Geometry check sheet. Reference: the model listing, model coordinates, mm. A direction names the side the tool comes from. Round coordinates to 2 decimals unless told otherwise and drop trailing zeros. Write each loop counter-clockwise with the first axis right and the second up, starting at its lowest first coordinate (ties: lowest second). Pieces come first, ordered by that corner, then holes. Notation, with made-up numbers: (-18, -13) -> (15, -13) arc R23 ccw to (15, 16) -> close; hole circle Ø3 at (-39, 32.25). An arc over 180 degrees is marked (long way). Use a Markdown table: item, result.
```python
from build123d import *

# Parameters (mm, degrees)
SKETCH1_W           = 85
SKETCH1_H           = 20
BOSS_EXTRUDE1_DEPTH = 5
CUT_EXTRUDE1_REACH  = 7
SKETCH2_W           = 8
SKETCH2_H           = 5.2


with BuildPart() as part:
    # Sketch1 → Boss-Extrude1 (new body)
    with BuildSketch(Plane.XY):
        with Locations((20.528766582, 10)):
            Rectangle(SKETCH1_W, SKETCH1_H)
    extrude(amount=BOSS_EXTRUDE1_DEPTH)

    # Sketch2 → Cut-Extrude1 (cut, up to next)
    with BuildSketch(Plane.XY.offset(5), mode=Mode.PRIVATE) as cut_extrude1_sk1:
        with Locations((-7.971233418, 4.6)):
            Rectangle(SKETCH2_W, SKETCH2_H)
    cut_extrude1_tool1 = extrude(cut_extrude1_sk1.sketch, amount=-CUT_EXTRUDE1_REACH, mode=Mode.PRIVATE) & part.part
    add(cut_extrude1_tool1.solids().sort_by_distance((-7.971233, 4.6, 5))[0], mode=Mode.SUBTRACT)
    # Sketch2 → Cut-Extrude1 (cut, up to next)
    with BuildSketch(Plane.XY.offset(5), mode=Mode.PRIVATE) as cut_extrude1_sk2:
        with Locations((11.028766582, 4.6)):
            Rectangle(SKETCH2_W, SKETCH2_H)
    cut_extrude1_tool2 = extrude(cut_extrude1_sk2.sketch, amount=-CUT_EXTRUDE1_REACH, mode=Mode.PRIVATE) & part.part
    add(cut_extrude1_tool2.solids().sort_by_distance((11.028767, 4.6, 5))[0], mode=Mode.SUBTRACT)
    # Sketch2 → Cut-Extrude1 (cut, up to next)
    with BuildSketch(Plane.XY.offset(5), mode=Mode.PRIVATE) as cut_extrude1_sk3:
        with Locations((30.028766582, 4.6)):
            Rectangle(SKETCH2_W, SKETCH2_H)
    cut_extrude1_tool3 = extrude(cut_extrude1_sk3.sketch, amount=-CUT_EXTRUDE1_REACH, mode=Mode.PRIVATE) & part.part
    add(cut_extrude1_tool3.solids().sort_by_distance((30.028767, 4.6, 5))[0], mode=Mode.SUBTRACT)
    # Sketch2 → Cut-Extrude1 (cut, up to next)
    with BuildSketch(Plane.XY.offset(5), mode=Mode.PRIVATE) as cut_extrude1_sk4:
        with Locations((49.028766582, 4.6)):
            Rectangle(SKETCH2_W, SKETCH2_H)
    cut_extrude1_tool4 = extrude(cut_extrude1_sk4.sketch, amount=-CUT_EXTRUDE1_REACH, mode=Mode.PRIVATE) & part.part
    add(cut_extrude1_tool4.solids().sort_by_distance((49.028767, 4.6, 5))[0], mode=Mode.SUBTRACT)


solid = part.part
```
(1) Section check B-B on x = 9. Record the cut outline in (y, z).
A:
| item | result |
|---|---|
| outline | (0, 0) -> (2, 0) -> (2, 5) -> (0, 5) -> close; (7.2, 0) -> (20, 0) -> (20, 5) -> (7.2, 5) -> close |
(2) Section check A-A on y = 3.75. Record the cut outline in (x, z).
A:
| item | result |
|---|---|
| outline | (-21.97, 0) -> (-11.97, 0) -> (-11.97, 5) -> (-21.97, 5) -> close; (-3.97, 0) -> (7.03, 0) -> (7.03, 5) -> (-3.97, 5) -> close; (15.03, 0) -> (26.03, 0) -> (26.03, 5) -> (15.03, 5) -> close; (34.03, 0) -> (45.03, 0) -> (45.03, 5) -> (34.03, 5) -> close; (53.03, 0) -> (63.03, 0) -> (63.03, 5) -> (53.03, 5) -> close |
(3) Section check C-C on z = 2.6. Record the cut outline in (x, y), plus the area to 3 significant figures.
A:
| item | result |
|---|---|
| outline | (-21.97, 0) -> (63.03, 0) -> (63.03, 20) -> (-21.97, 20) -> close; hole (-11.97, 2) -> (-3.97, 2) -> (-3.97, 7.2) -> (-11.97, 7.2) -> close; hole (7.03, 2) -> (15.03, 2) -> (15.03, 7.2) -> (7.03, 7.2) -> close; hole (26.03, 2) -> (34.03, 2) -> (34.03, 7.2) -> (26.03, 7.2) -> close; hole (45.03, 2) -> (53.03, 2) -> (53.03, 7.2) -> (45.03, 7.2) -> close |
| area | 1,530 mm2 |
(4) Thickness scan on line 1 (X direction, y = 6, z = 2.05); line 2 (Y direction, x = -10, z = 0.9). Record the ranges inside material, lowest first.
A:
| item | result |
|---|---|
| line 1 | x = -21.97 to -11.97, -3.97 to 7.03, 15.03 to 26.03, 34.03 to 45.03, 53.03 to 63.03 |
| line 2 | y = 0 to 2, 7.2 to 20 |
(5) Release check for a two-part mould opening along Y. For faces 1 (the face through (-21.971, 10, 2)), 2 (the face through (20, 0, 2)), 3 (the face through (30, 2, 3)) record: +Y half, -Y half, draft (parallel to the pull), parting line (faces both ways), or undercut.
A:
| item | result |
|---|---|
| face 1 | draft |
| face 2 | -Y half |
| face 3 | undercut |
(6) Access from +Z, -Z, +X, -X, +Y, -Y to the whole of each face (thin tool, end or side, straight path). Record for faces 4 (the face through (11, 7.2, 3)), 5 (the face through (20, 10, 5)).
A:
| item | result |
|---|---|
| face 4 | +Z, -Z |
| face 5 | +Z, +X, -X, +Y, -Y |
